For this review, take the finished solid that the model builds, in its own axes (mm). Coordinates: 2 decimals unless noted, no trailing zeros. Write each loop counter-clockwise with the first axis right and the second up, starting at its lowest first coordinate (ties: lowest second). Pieces come first, ordered by that corner, then holes. Notation, with made-up numbers: (-10, -6.75) - (44, -6.75) arc R29 ccw to (44, 13.25) - close; hole circle Ø6 at (-34, -9.5). An arc over 180 degrees is marked (long way). Write each question's results on one line, items separated by ' | '.
from build123d import *

# Parameters (mm, degrees)
SKETCH1_R           = 2.1082
SKETCH1_R_2         = 10.287
BOSS_EXTRUDE1_DEPTH = 1.5875


with BuildPart() as part:
    # Sketch1 → Boss-Extrude1 (new body)
    with BuildSketch(Plane.XY.offset(16.51)):
        with BuildLine():
            Line((13.6525, -15.397931679), (13.6525, 15.397931679))
            ThreePointArc((13.6525, 15.397931679), (10.678479761, 19.811858094), (5.470769231, 18.71308887))
            ThreePointArc((5.470769231, 18.71308887), (0, 16.397340374), (-5.470769231, 18.71308887))
            ThreePointArc((-5.470769231, 18.71308887), (-10.678479761, 19.811858094), (-13.6525, 15.397931679))
            Line((-13.6525, 15.397931679), (-13.6525, -15.397931679))
            ThreePointArc((-13.6525, -15.397931679), (-10.678479761, -19.811858094), (-5.470769231, -18.71308887))
            ThreePointArc((-5.470769231, -18.71308887), (0, -16.397340374), (5.470769231, -18.71308887))
            ThreePointArc((5.470769231, -18.71308887), (10.678479761, -19.811858094), (13.6525, -15.397931679))
        make_face()
        with Locations((8.89, -15.397931679)):
            Circle(SKETCH1_R, mode=Mode.SUBTRACT)
        with Locations((-8.89, -15.397931679)):
            Circle(SKETCH1_R, mode=Mode.SUBTRACT)
        Circle(SKETCH1_R_2, mode=Mode.SUBTRACT)
        with Locations((8.89, 15.397931679)):
            Circle(SKETCH1_R, mode=Mode.SUBTRACT)
        with Locations((-8.89, 15.397931679)):
            Circle(SKETCH1_R, mode=Mode.SUBTRACT)
    extrude(amount=BOSS_EXTRUDE1_DEPTH)


solid = part.part
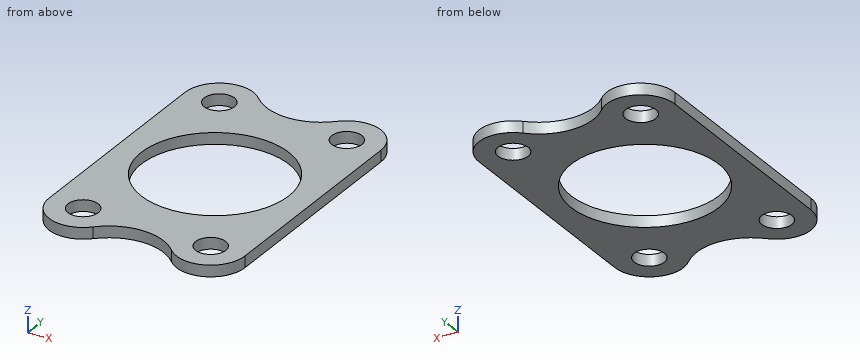
Q1. Take a section at D-D on x = 8.75. State the section outline as (y, z) points.
Results found:
outline: (-20.16, 16.51) - (-17.5, 16.51) - (-17.5, 18.1) - (-20.16, 18.1) - close; (-13.29, 16.51) - (-5.41, 16.51) - (-5.41, 18.1) - (-13.29, 18.1) - close; (5.41, 16.51) - (13.29, 16.51) - (13.29, 18.1) - (5.41, 18.1) - close; (17.5, 16.51) - (20.16, 16.51) - (20.16, 18.1) - (17.5, 18.1) - close
Q2. Take a section at C-C on z = 17.45. State the section outline as (x, y) points (1 decimal).
Results found:
outline: (-13.7, -15.4) arc R4.8 ccw to (-5.5, -18.7) arc R7.6 cw to (5.5, -18.7) arc R4.8 ccw to (13.7, -15.4) - (13.7, 15.4) arc R4.8 ccw to (5.5, 18.7) arc R7.6 cw to (-5.5, 18.7) arc R4.8 ccw to (-13.7, 15.4) - close; hole circle Ø4.2 at (-8.9, -15.4); hole circle Ø4.2 at (-8.9, 15.4); hole circle Ø20.6 at (0, 0); hole circle Ø4.2 at (8.9, -15.4); hole circle Ø4.2 at (8.9, 15.4)
Q3. Wall thickness on line 1 along Y through (x, z) = (7.75, 17.9); line 2 along X through (y, z) = (13.5, 17.85); line 3 along Y through (x, z) = (-8.89, 17.05): over which ranges is each line inside the solid? List them lowest first. Write a range as from..to.
Results found:
line 1: -20.02..-17.17, -13.62..-6.76, 6.76..13.62, 17.17..20.02 | line 2: -13.65..-9.81, -7.97..7.97, 9.81..13.65 | line 3: -20.16..-17.51, -13.29..-5.18, 5.18..13.29, 17.51..20.16
Q4. Take a section at B-B on y = 0. State the section outline as (x, z) points, plus the area to 3 significant figures.
Results found:
outline: (-13.65, 16.51) - (-10.29, 16.51) - (-10.29, 18.1) - (-13.65, 18.1) - close; (10.29, 16.51) - (13.65, 16.51) - (13.65, 18.1) - (10.29, 18.1) - close | area: 10.7 mm2
Q5. For pin 1 (3.5 mm diameter, centred on x = -8.89, y = 15.4, fed in from -Z), flat-tipped, find the tip position at first contact; note if it passes through.
Results found:
pin 1: through
Q6. Take a section at A-A on x = 0. State the section outline as (y, z) points.
Results found:
outline: (-16.4, 16.51) - (-10.29, 16.51) - (-10.29, 18.1) - (-16.4, 18.1) - close; (10.29, 16.51) - (16.4, 16.51) - (16.4, 18.1) - (10.29, 18.1) - close
